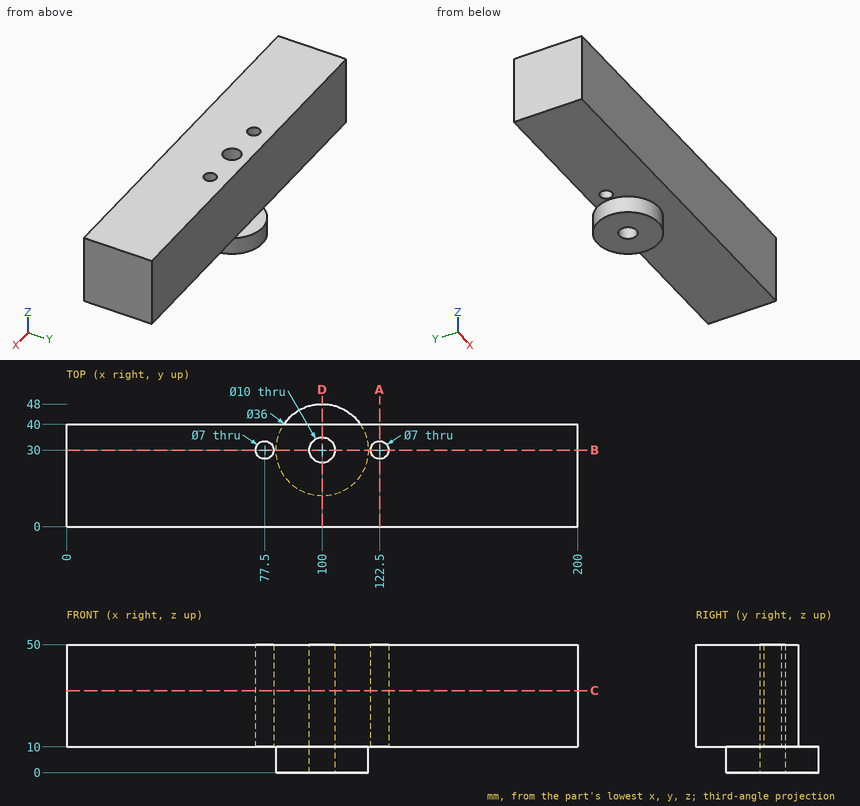
Study the drawing (mm; zero at the part's minimum x, y, z) and answer. Give positions to 0.01 mm unless a question says otherwise; leave off trailing zeros. Write each loop counter-clockwise with the first axis right and the second up, starting at its lowest first coordinate (ties: lowest second). Pieces come first, ordered by that corner, then holes. Notation, with made-up numbers: (52.5, 45) -> (69.5, 45) arc R15 ccw to (69.5, 63) -> close; hole circle Ø4 at (-4, 85.25). An arc over 180 degrees is marked (long way). Answer as a JSON object with one key per item and string values. Group by question number.
1) Consider L1, parallel to Y at x = 77.5, z = 37; L2, parallel to Z at x = 94, y = 3; L3, parallel to Y at x = 41, z = 31. Determine where each line is inside the solid, lowest interval first. Write a range as from..to.
2) Find section C-C (z = 32). Write down the section's boundary in (x, y), and give its area (3 significant figures).
3) Each of these flat-tipped pins is pushed along its axis until it touches: P1, Ø8, axis at x = 62, y = 23.5, coming from the -Z side; P2, Ø2.5, axis at x = 96.5, y = 43, coming from the +Z side; P3, Ø9, axis at x = 100, y = 30, coming from the -Z side; P4, Ø1.5, axis at x = 159.5, z = 37.5, coming from the +Y side. Where does it stop, or does it pass through?
4) Find section D-D (x = 100). Write down the section's boundary in (y, z), and give its area (3 significant figures).
5) Find section B-B (y = 30). Write down the section's boundary in (x, z), and give its area (3 significant figures).
6) Find section A-A (x = 122.5). Write down the section's boundary in (y, z), and give its area (3 significant figures).
Values follow:
{
 "1": {"L1": "y = 0..26.5, 33.5..40", "L2": "z = 10..50", "L3": "y = 0..40"},
 "2": {"outline": "(0, 0) -> (200, 0) -> (200, 40) -> (0, 40) -> close; hole circle Ø7 at (77.5, 30); hole circle Ø10 at (100, 30); hole circle Ø7 at (122.5, 30)", "area": "7,840 mm2"},
 "3": {"P1": "stops at z = 10", "P2": "stops at z = 10", "P3": "passes through", "P4": "stops at y = 40"},
 "4": {"outline": "(0, 10) -> (12, 10) -> (12, 0) -> (25, 0) -> (25, 50) -> (0, 50) -> close; (35, 0) -> (48, 0) -> (48, 10) -> (40, 10) -> (40, 50) -> (35, 50) -> close", "area": "1,460 mm2"},
 "5": {"outline": "(0, 10) -> (74, 10) -> (74, 50) -> (0, 50) -> close; (81, 10) -> (82, 10) -> (82, 0) -> (95, 0) -> (95, 50) -> (81, 50) -> close; (105, 0) -> (118, 0) -> (118, 10) -> (119, 10) -> (119, 50) -> (105, 50) -> close; (126, 10) -> (200, 10) -> (200, 50) -> (126, 50) -> close", "area": "7,300 mm2"},
 "6": {"outline": "(0, 10) -> (26.5, 10) -> (26.5, 50) -> (0, 50) -> close; (33.5, 10) -> (40, 10) -> (40, 50) -> (33.5, 50) -> close", "area": "1,320 mm2"}
}
